Geometry check sheet. Reference: the model listing, model coordinates, mm. Round coordinates to 2 decimals unless told otherwise and drop trailing zeros. Loops run counter-clockwise (first coordinate to the right, second up) from the corner with the lowest first, then second, coordinate; pieces in that order, holes last. Notation, with made-up numbers: (28, -33.75) - (37, -33.75) arc R14 ccw to (37, -27.75) - close; hole circle Ø3 at (9.25, 83.5). An arc over 180 degrees is marked (long way). Answer as CSV lines item,"result". Start each with the question number.
1) Cross-section at A-A on x = 40. Record the boundary of the cut face in (y, z), and give its area (3 significant figures).
2) Cross-section at B-B on z = 10. Record the boundary of the cut face in (x, y).
3) Thickness scan on line 1 along X through (y, z) = (3.2, 10). Record the ranges inside material, lowest first.
4) Draft check along X on faces 1 (the flat face through (-79, 3, 0)), 2 (the flat face through (-1, 0, 0)), 3 (the cylindrical face through (42.53, 2.46, 11.61)), 4 (the cylindrical face through (-37.47, 2.46, 11.61)). Enter one of: released by +X, released by -X, zero draft, split by the parting line, or undercut.
from build123d import *

# Parameters (mm, degrees)
SKIZZE1_W                       = 160
SKIZZE1_H                       = 50
SKIZZE1_R                       = 3
AUFSATZ_LINEAR_AUSTRAGEN1_DEPTH = 5
SKIZZE2_W                       = 160
SKIZZE2_H                       = 50
SKIZZE2_W_2                     = 158
SKIZZE2_H_2                     = 48
SCHNITT_LINEAR_AUSTRAGEN1_DEPTH = 10


with BuildPart() as part:
    # Skizze1 → Aufsatz-Linear austragen1 (new body)
    with BuildSketch(Plane(origin=(0, 0, 0), x_dir=(1, 0, 0), z_dir=(0, 1, 0))):
        Rectangle(SKIZZE1_W, SKIZZE1_H)
        with Locations(Location((-40, 10, 0), (0, 0, 270))):
            Circle(SKIZZE1_R, mode=Mode.SUBTRACT)
        with Locations(Location((-40, -10, 0), (0, 0, 270))):
            Circle(SKIZZE1_R, mode=Mode.SUBTRACT)
        with Locations(Location((40, 10, 0), (0, 0, 270))):
            Circle(SKIZZE1_R, mode=Mode.SUBTRACT)
        with Locations(Location((40, -10, 0), (0, 0, 270))):
            Circle(SKIZZE1_R, mode=Mode.SUBTRACT)
    extrude(amount=AUFSATZ_LINEAR_AUSTRAGEN1_DEPTH)

    # Skizze2 → Schnitt-Linear austragen1 (cut)
    with BuildSketch(Plane(origin=(0, 5, 0), x_dir=(1, 0, 0), z_dir=(0, 1, 0))):
        Rectangle(SKIZZE2_W, SKIZZE2_H)
        Rectangle(SKIZZE2_W_2, SKIZZE2_H_2, mode=Mode.SUBTRACT)
    extrude(amount=-SCHNITT_LINEAR_AUSTRAGEN1_DEPTH, mode=Mode.SUBTRACT)


solid = part.part
Answer block:
1,outline,"(0, -24) - (5, -24) - (5, -13) - (0, -13) - close; (0, -7) - (5, -7) - (5, 7) - (0, 7) - close; (0, 13) - (5, 13) - (5, 24) - (0, 24) - close"
1,area,"180 mm^2"
2,outline,"(-79, 0) - (-43, 0) - (-43, 5) - (-79, 5) - close; (-37, 0) - (37, 0) - (37, 5) - (-37, 5) - close; (43, 0) - (79, 0) - (79, 5) - (43, 5) - close"
3,line 1,"x = -79 to -43, -37 to 37, 43 to 79"
4,face 1,"released by -X"
4,face 2,"zero draft"
4,face 3,"undercut"
4,face 4,"undercut"
